Check sheet for the modelled part. Datum: model origin and axes. Units: mm. A direction names the side the tool comes from. Give positions to 0.01 mm unless a question says otherwise; leave off trailing zeros. Write each loop counter-clockwise with the first axis right and the second up, starting at its lowest first coordinate (ties: lowest second). Pieces come first, ordered by that corner, then holes. Notation, with made-up numbers: (-5.5, 68.25) -> (18.5, 68.25) arc R31 ccw to (18.5, 107.25) -> close; hole circle Ø2 at (0, 86). An arc over 180 degrees is marked (long way). Return JSON: item names as keys, results as strings.
Autodesk Inventor part; units mm, degrees
ref_plane "YZ Plane" through (0, 0, 0) normal (1, 0, 0) x (0, 1, 0)
ref_plane "XZ Plane" through (0, 0, 0) normal (0, 1, 0) x (-1, 0, 0)
ref_plane "XY Plane" through (0, 0, 0) normal (0, 0, 1) x (1, 0, 0)
ref_plane "РабПлоскость1" through (0, 0, 0) normal (0, 0, 1) x (1, 0, 0)
sketch "Эскиз1" plane through (0, 0, 0) normal (0, 0, 1) x (1, 0, 0)
  circle A0 centre (-141.8, -95) radius 4
  circle A1 centre (-94.4, -95) radius 4
  circle A2 centre (-47, -95) radius 4
  circle A3 centre (0.4, -95) radius 4
  circle A4 centre (47.8, -95) radius 4
  circle A5 centre (95.2, -95) radius 4
  circle A6 centre (142.6, -95) radius 4
  circle A7 centre (189.4425, -146.4995) radius 4
  circle A8 centre (189.4425, -194.4995) radius 4
  circle A9 centre (189.4425, -242.4995) radius 4
  circle A10 centre (189.4425, -290.4995) radius 4
  circle A11 centre (165.7163, -328.1346) radius 4
  circle A12 centre (117.9209, -330) radius 4
  circle A13 centre (69.9209, -330) radius 4
  circle A14 centre (21.9209, -330) radius 4
  circle A15 centre (-26.0791, -330) radius 4
  circle A16 centre (-74.0791, -330) radius 4
  circle A17 centre (-122.0791, -330) radius 4
  circle A18 centre (-169.6605, -327.0042) radius 4
  circle A19 centre (-190.486, -287.3914) radius 4
  circle A20 centre (-190.4444, -239.3914) radius 4
  circle A21 centre (-190.4029, -191.3914) radius 4
  circle A22 centre (-190.3613, -143.3914) radius 4
  circle A23 centre (-190.3198, -95.3914) radius 4
  circle A24 centre (-190.2782, -47.3914) radius 4
  circle A25 centre (-190.2367, 0.6085) radius 4
  circle A26 centre (-190.1952, 48.6085) radius 4
  circle A27 centre (-190.1536, 96.6085) radius 4
  circle A28 centre (-190.1121, 144.6085) radius 4
  circle A29 centre (-190.0705, 192.6085) radius 4
  circle A30 centre (-190.029, 240.6084) radius 4
  circle A31 centre (-189.9874, 288.6084) radius 4
  circle A32 centre (-168.0002, 327.4583) radius 4
  circle A33 centre (-120.3208, 329.9395) radius 4
  circle A34 centre (-72.3208, 329.8979) radius 4
  circle A35 centre (-24.3209, 329.8564) radius 4
  circle A36 centre (23.6791, 329.8148) radius 4
  circle A37 centre (71.6791, 329.7733) radius 4
  circle A38 centre (119.6791, 329.7317) radius 4
  circle A39 centre (167.4036, 327.4296) radius 4
  circle A40 centre (190, 289) radius 4
  circle A41 centre (190, 241) radius 4
  circle A42 centre (190, 193) radius 4
  circle A43 centre (190, 145) radius 4
  circle A44 centre (190, 97) radius 4
  circle A45 centre (190, 49) radius 4
  circle A46 centre (190, 1) radius 4
  circle A47 centre (190, -47) radius 4
  circle A48 centre (190, -95) radius 4
  line L0 (200, 300) -> (200, -300)
  arc A49 (200, 300) -> (160, 340) centre (160, 300) ccw
  line L1 (-160, 340) -> (160, 340)
  arc A50 (-160, 340) -> (-200, 300) centre (-160, 300) ccw
  line L2 (-200, -300) -> (-200, 300)
  arc A51 (-200, -300) -> (-160, -340) centre (-160, -300) ccw
  line L3 (160, -340) -> (-160, -340)
  arc A52 (160, -340) -> (200, -300) centre (160, -300) ccw
  line L4 (180, -110) -> (-180, -110)
  line L5 (180, -290) -> (180, -110)
  arc A53 (150, -320) -> (180, -290) centre (150, -290) ccw
  line L6 (-150, -320) -> (150, -320)
  arc A54 (-180, -290) -> (-150, -320) centre (-150, -290) ccw
  line L7 (-180, -110) -> (-180, -290)
  line L8 (180, -80) -> (180, 290)
  line L9 (-180, -80) -> (180, -80)
  line L10 (-180, 290) -> (-180, -80)
  arc A55 (-150, 320) -> (-180, 290) centre (-150, 290) ccw
  line L11 (150, 320) -> (-150, 320)
  arc A56 (180, 290) -> (150, 320) centre (150, 290) ccw
  point P0 (0, 0)
extrude "Выдавливание1" add sketch "Эскиз1" along normal blind 2
properties part number "Прокладка крышки фонаря 2" material "Алюминий 6061"
(1) Cross-section at A-A on y = -171.5. Enter the section's corners in (x, z), then the cut area to 3 significant figures.
Reply:
{"outline": "(-200, 0) -> (-180, 0) -> (-180, 2) -> (-200, 2) -> close; (180, 0) -> (200, 0) -> (200, 2) -> (180, 2) -> close", "area": "80.0 mm^2"}
(2) Set-up check for faces 4 (the cylindrical face through (-188.594, 327.972, 0.986)), 5 (the cylindrical face through (-170.979, -311.445, 0.986)): record each of +Z, -Z, +X, -X, +Y, -Y from which the full face is reachable in a straight line by a thin tool's end or side.
Reply:
{"face 4": "+Z, -Z, -X, +Y", "face 5": "+Z, -Z"}
(3) Depth check by flat-ended pin: pin 1 Ø7 at (x, y) = (189.44, -194.5) entering from +Z. Enter the tip coordinate at first touch or a pass-through.
Reply:
{"pin 1": "through"}
(4) Cross-section at B-B on z = 0.9. State how many separate pieces and enclosed holes the cut face has, then the cut area to 3 significant figures.
Reply:
{"separate pieces": "1", "enclosed holes": "51", "area": "49,300 mm^2"}
(5) Release check for a two-part mould opening along X. For faces 1 (the cylindrical face through (188.594, -327.972, 0.986)), 2 (the flat face through (-1, -99, 2)), 3 (the cylindrical face through (171.445, -310.979, 0.986)) record: pulls with the +X half, pulls with the -X half, needs draft (parallel to the pull), parting line crosses it, or undercut.
Reply:
{"face 1": "pulls with the +X half", "face 2": "needs draft", "face 3": "undercut"}
(6) Thickness scan on L1, parallel to Y at x = -1.5, z = 1.5; L2, parallel to Y at x = 60.5, z = 1.5; L3, parallel to X at y = -24, z = 1.75. Record the ranges inside material, lowest first.
Reply:
{"L1": "-340 to -320, -110 to -98.52, -91.48 to -80, 320 to 340", "L2": "-340 to -320, -110 to -80, 320 to 340", "L3": "-200 to -180, 180 to 200"}
